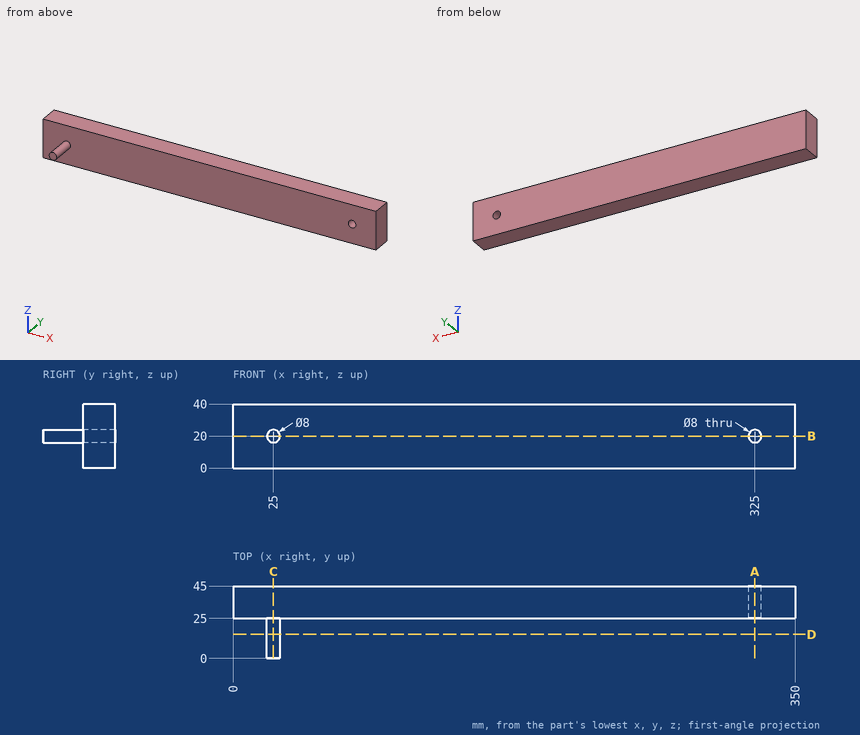
Geometry: see drawing. Coordinates: mm, zero at the bounding-box minimum. Round coordinates to 2 decimals unless told otherwise and drop trailing zeros. Loops run counter-clockwise (first coordinate to the right, second up) from the corner with the lowest first, then second, coordinate; pieces in that order, holes last. Notation, with made-up numbers: (-24, 37) -> (29, 37) arc R15 cw to (29, 44) -> close; hole circle Ø9 at (36, 47). An arc over 180 degrees is marked (long way). Use one line per item in the form item = value. Start each with the question number.
Item 1: Section query B-B on z = 20. Return the cut outline in (x, y), then the cut area to 3 significant figures.
Item 2: Section query C-C on x = 25. Return the cut outline in (y, z), then the cut area to 3 significant figures.
Item 3: Section query D-D on y = 15. Return the cut outline in (x, z).
Item 4: Contact query for flat-ended pins moving along their axis: pin 1 Ø10 at (y, z) = (30.5, 21) entering from -X; pin 2 Ø3 at (x, z) = (309, 33.5) entering from -Y. Output: stop coordinate, or through.
Item 5: Section query A-A on x = 325. Return the cut outline in (y, z), then the cut area to 3 significant figures.
Item 6: Material intervals for L1, parallel to Z at x = 325, y = 31; L2, parallel to Y at x = 81, z = 26, sorted ascending. Write a range as from..to.
Ans:
q1.outline = (0, 25) -> (21, 25) -> (21, 0) -> (29, 0) -> (29, 25) -> (321, 25) -> (321, 45) -> (0, 45) -> close; (329, 25) -> (350, 25) -> (350, 45) -> (329, 45) -> close
q1.area = 7,040 mm^2
q2.outline = (0, 16) -> (25, 16) -> (25, 0) -> (45, 0) -> (45, 40) -> (25, 40) -> (25, 24) -> (0, 24) -> close
q2.area = 1,000 mm^2
q3.outline = circle Ø8 at (25, 20)
q4.pin_1 = 0
q4.pin_2 = 25
q5.outline = (25, 0) -> (45, 0) -> (45, 16) -> (25, 16) -> close; (25, 24) -> (45, 24) -> (45, 40) -> (25, 40) -> close
q5.area = 640 mm^2
q6.L1 = 0..16, 24..40
q6.L2 = 25..45
